Here's the drawing with two shaded views (mm, measured from the low corner). I have some questions. A direction names the side the tool comes from. Coordinates: 2 decimals unless noted, no trailing zeros. Loops run counter-clockwise (first coordinate to the right, second up) from the corner with the lowest first, then second, coordinate; pieces in that order, holes last. Notation, with made-up numbers: (43.25, 73.25) -> (60.25, 73.25) arc R16 ccw to (60.25, 84.25) -> close; hole circle Ø9 at (89.5, 55). An arc over 180 degrees is marked (long way). Answer as a JSON object with one key per item and string values. Group by question number.
1) I want a section at A-A (y = 53). Write out the boundary of the cut face in (x, z) (1 decimal).
2) I want a section at D-D (x = 16). Write out the boundary of the cut face in (y, z), then the cut area to 3 significant figures.
3) I want a section at C-C (z = 14.25). Write out the boundary of the cut face in (x, y) (1 decimal).
4) I need wall thicknesses on probe 1 along Z at (x, y) = (10.5, 127.5); probe 2 along Z at (x, y) = (69, 25.5); probe 3 along Y at (x, z) = (17, 6.5). Which ranges of each line are inside material? Lowest first, please. Write a range as [from, to].
5) I'm going to push flat-ended pins straight in: pin 1 (6 mm diameter, centred on x = 80.5, y = 45, fed in from -Z); pin 2 (8.5 mm diameter, centred on x = 13, y = 96, fed in from -Z); pin 3 (1.9 mm diameter, centred on y = 129.5, z = 21.5, fed in from +X). Where does each tip first touch, or does it pass through?
6) Which directions (+Z, -Z, +X, -X, +Y, -Y) give clear straight access to the entire face, cutting with the end or side of a thin tool? Please do the marked faces 1, 2 and 3.
7) I want a section at B-B (x = 62.5). Write out the boundary of the cut face in (y, z), then the cut area to 3 significant figures.
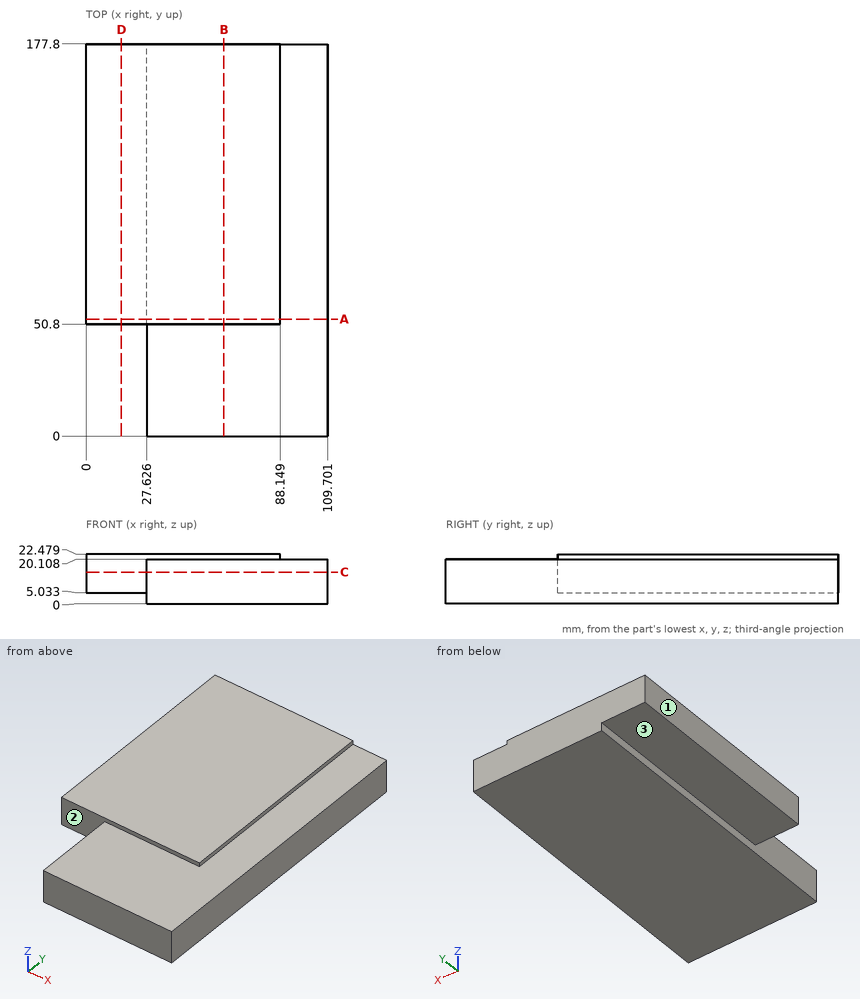
Determined:
{
 "1": {"outline": "(0, 5) -> (27.6, 5) -> (27.6, 0) -> (109.7, 0) -> (109.7, 20.1) -> (88.1, 20.1) -> (88.1, 22.5) -> (0, 22.5) -> close"},
 "2": {"outline": "(50.8, 5.03) -> (177.8, 5.03) -> (177.8, 22.48) -> (50.8, 22.48) -> close", "area": "2,220 mm^2"},
 "3": {"outline": "(0, 50.8) -> (27.6, 50.8) -> (27.6, 0) -> (109.7, 0) -> (109.7, 177.8) -> (0, 177.8) -> close"},
 "4": {"probe 1": "[5.03, 22.48]", "probe 2": "[0, 20.11]", "probe 3": "[50.8, 177.8]"},
 "5": {"pin 1": "z = 0", "pin 2": "z = 5.03", "pin 3": "x = 88.15"},
 "6": {"face 1": "+Z, -Z, -X, +Y, -Y", "face 2": "+Z, -X, -Y", "face 3": "-Z, -X, +Y, -Y"},
 "7": {"outline": "(0, 0) -> (177.8, 0) -> (177.8, 22.48) -> (50.8, 22.48) -> (50.8, 20.11) -> (0, 20.11) -> close", "area": "3,880 mm^2"}
}
